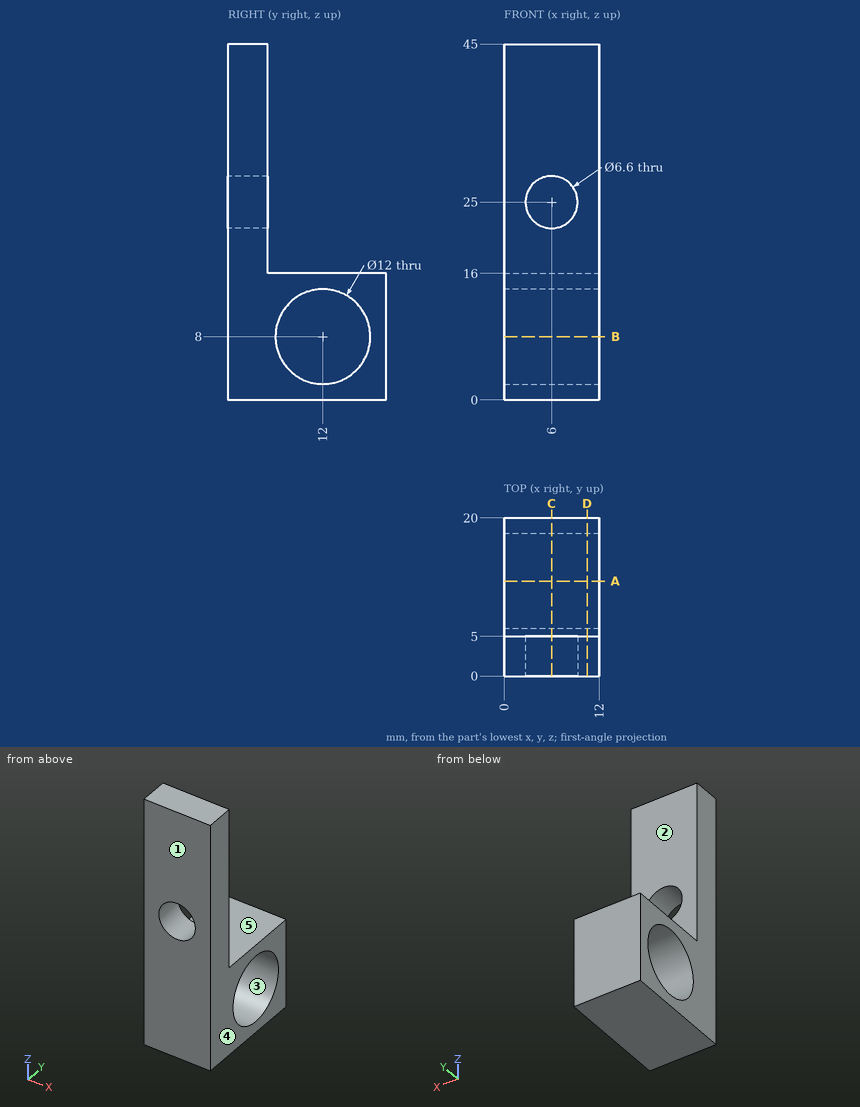
For this review, use the dimensioned drawing (mm, ordinates from the lowest corner) and the shaded views. A direction names the side the tool comes from. Give positions to 0.01 mm unless a question says otherwise; leave off trailing zeros. Write each loop counter-clockwise with the first axis right and the second up, starting at its lowest first coordinate (ties: lowest second). Pieces come first, ordered by that corner, then holes.
(1) To check wall thickness, follow L1, parallel to Y at x = 3.75, z = 8; L2, parallel to Z at x = 6, y = 1.6; L3, parallel to Y at x = 2.5, z = 29. State the ranges of each line that lie inside material, in increasing order.
(2) Tool access review of the marked faces 1 and 2: name each direction out of +Z, -Z, +X, -X, +Y, -Y from which nothing blocks a thin tool from reaching the whole face with its end or side.
(3) Consider section A-A, the plane y = 12. Give the boundary of the cut face in (x, z), and give its area (3 significant figures).
(4) Consider section C-C, the plane x = 6. Give the boundary of the cut face in (y, z), and give its area (3 significant figures).
(5) The part is to be moulded in two halves that separate along Z. For the marked faces 3, 4 and 5, say which applies: released by +Z, released by -Z, zero draft, split by the parting line, or undercut.
(6) For P1, Ø5, axis at x = 8, z = 33, coming from the +Y side; P2, Ø4, axis at x = 6, z = 25, coming from the +Y side, all flat-tipped, find the tip position at first contact; note any pin that passes through.
(7) Consider section B-B, the plane z = 8. Give the boundary of the cut face in (x, y), and give its area (3 significant figures).
(8) Consider section D-D, the plane x = 10.5. Give the boundary of the cut face in (y, z), and give its area (3 significant figures).
Returned:
1. L1: y = 0 to 6, 18 to 20
1. L2: z = 0 to 21.7, 28.3 to 45
1. L3: y = 0 to 5
2. face 1: +Z, -Z, +X, -X, -Y
2. face 2: +Z, +X, -X, +Y
3. outline: (0, 0) - (12, 0) - (12, 2) - (0, 2) - close; (0, 14) - (12, 14) - (12, 16) - (0, 16) - close
3. area: 48.0 mm2
4. outline: (0, 0) - (20, 0) - (20, 16) - (5, 16) - (5, 21.7) - (0, 21.7) - close; (0, 28.3) - (5, 28.3) - (5, 45) - (0, 45) - close; hole circle Ø12 at (12, 8)
4. area: 319 mm2
5. face 3: undercut
5. face 4: zero draft
5. face 5: released by +Z
6. P1: stops at y = 5
6. P2: passes through
7. outline: (0, 0) - (12, 0) - (12, 6) - (0, 6) - close; (0, 18) - (12, 18) - (12, 20) - (0, 20) - close
7. area: 96.0 mm2
8. outline: (0, 0) - (20, 0) - (20, 16) - (5, 16) - (5, 45) - (0, 45) - close; hole circle Ø12 at (12, 8)
8. area: 352 mm2
